Design review of the part built by this model. Coordinates are the model's own, in mm. A direction names the side the tool comes from. Give positions to 0.01 mm unless a question says otherwise; leave off trailing zeros. Loops run counter-clockwise (first coordinate to the right, second up) from the corner with the lowest first, then second, coordinate; pieces in that order, holes last. Notation, with made-up numbers: M 3.25,71.5 L 17.25,71.5 A32 ccw 17.25,107.5 Z; hole C -1,8 d7. An arc over 180 degrees is marked long. Use a Markdown table: item, result. Add a question column.
(1) Add section A-A, the plane x = 186. Give the boundary of the cut face in (y, z).
(2) Insertion check: pin 1 Ø1.5 at (x, y) = (199.5, -120.5) entering from +Z; pin 2 Ø5.5 at (x, z) = (2.5, -28.5) entering from +Y; pin 3 Ø1.5 at (x, y) = (51.5, -143) entering from +Z; pin 4 Ø6 at (y, z) = (-230, 15) entering from -X. Each pin has a flat end and moves straight along its axis. Give the tip position at first contact, or say it passes through.
(3) For faces 1 (the face through (138, -46.338, -1)), 2 (the face through (152, -41.338, -1)), list the 3-axis set-ups (+Z, -Z, +X, -X, +Y, -Y) from which the entire face can be reached by the end or side of a thin tool; tool diameter is ignored.
(4) For probe 1 along X at (y, z) = (-54.5, -0.5); probe 2 along Y at (x, z) = (119.5, -11.5); probe 3 along Y at (x, z) = (268, -5), list the stretches that pass through material, from the lowest coordinate up.
(5) Add section C-C, the plane y = -186.5. Give the boundary of the cut face in (x, z), then the cut area to 3 significant figures.
(6) Draft analysis for pull direction X (two halves, no side actions). For faces 3 (the face through (300, -204, -9)), 4 (the face through (147.9, -44.345, -22.148)), 5 (the face through (0, -204, -9)), 6 (the face through (275, -204, -11)), state which applies: pulls with the +X half, pulls with the -X half, needs draft (parallel to the pull), parting line crosses it, or undercut.
(7) Add section B-B, the plane y = -273.5. Give the boundary of the cut face in (x, z), then the cut area to 3 significant figures.
```python
from build123d import *

# Parameters (mm, degrees)
F1_DEPTH = 300
F2_T     = -5
F4_DEPTH = 25
F7_DEPTH = 5
F9_DEPTH = 300


# Not quite as in the source:
# - a feature of the source that left no trace in its solid (it failed there, or was rolled back) is left out
# - a feature names something its author has since deleted; it is built from what else it names


with BuildPart() as f1:
    # F0 (on Right) → F1 (new body)
    with BuildSketch(Plane.YZ):
        with BuildLine():
            ThreePointArc((-361.3383226016, -15), (-358.4093904135, -22.0710678119), (-351.3383226016, -25))
            Line((-351.3383226016, -25), (-51.3383226016, -25))
            ThreePointArc((-51.3383226016, -25), (-44.2672547897, -22.0710678119), (-41.3383226016, -15))
            Line((-41.3383226016, -15), (-41.3383226016, 13.3530771738))
            ThreePointArc((-41.3383226016, 13.3530771738), (-44.538361228, 20.6852341086), (-52.0904276652, 23.3247539622))
            Line((-52.0904276652, 23.3247539622), (-352.0904276652, 0.6975144458))
            ThreePointArc((-352.0904276652, 0.6975144458), (-358.6704795365, -2.474200969), (-361.3383226016, -9.2741623426))
            Line((-361.3383226016, -9.2741623426), (-361.3383226016, -15))
        make_face()
    extrude(amount=F1_DEPTH)

    # F2: a shell. OpenCascade refuses it in one call, so the cavity is built on its own and cut out:
    # the body offset inwards by the wall thickness, plus a prism from it out through each open face.
    f2_core = offset(f1.part, amount=F2_T, mode=Mode.PRIVATE)
    f2_exits = [f2_core.faces().sort_by_distance(p)[0] for p in [
        (150, -201.338323, -20),
    ]]
    add(f2_core, mode=Mode.SUBTRACT)
    extrude(f2_exits, amount=-F2_T, mode=Mode.SUBTRACT)

    # F4 (add): a face of the model
    f4_faces = [f1.faces().sort_by_distance(p)[0] for p in [
        (300, -183.9481701293, -5.8146709921),
    ]]
    extrude(f4_faces, amount=-F4_DEPTH)

    # F7 (add): faces of the model
    f7_faces = [f1.faces().sort_by_distance(p)[0] for p in [
        (2.5, -201.3383226016, -25),
        (287.5, -201.3383226016, -25),
    ]]
    extrude(f7_faces, amount=F7_DEPTH)

    # F0 (on Right) → F9 (cut)
    with BuildSketch(Plane.YZ):
        with BuildLine():
            ThreePointArc((-361.3383226016, -15), (-358.4093904135, -22.0710678119), (-351.3383226016, -25))
            Line((-351.3383226016, -25), (-51.3383226016, -25))
            ThreePointArc((-51.3383226016, -25), (-44.2672547897, -22.0710678119), (-41.3383226016, -15))
            Line((-41.3383226016, -15), (-41.3383226016, 13.3530771738))
            ThreePointArc((-41.3383226016, 13.3530771738), (-44.538361228, 20.6852341086), (-52.0904276652, 23.3247539622))
            Line((-52.0904276652, 23.3247539622), (-352.0904276652, 0.6975144458))
            ThreePointArc((-352.0904276652, 0.6975144458), (-358.6704795365, -2.474200969), (-361.3383226016, -9.2741623426))
            Line((-361.3383226016, -9.2741623426), (-361.3383226016, -15))
        make_face()
    extrude(amount=-F9_DEPTH, mode=Mode.SUBTRACT)


solid = f1.part
```
Established:
| question | item | result |
|---|---|---|
| 1 | outline | M -361.34,-15 A10 ccw -351.34,-25 L -351.34,-20 A5 cw -356.34,-15 L -356.34,-9.27 A5 cw -351.71,-4.29 L -51.71,18.34 A5 cw -46.34,13.35 L -46.34,-15 A5 cw -51.34,-20 L -51.34,-25 A10 ccw -41.34,-15 L -41.34,13.35 A10 ccw -52.09,23.32 L -352.09,0.7 A10 ccw -361.34,-9.27 Z |
| 2 | pin 1 | z = 18.22 |
| 2 | pin 2 | y = -51.34 |
| 2 | pin 3 | z = 16.52 |
| 2 | pin 4 | through |
| 3 | face 1 | none |
| 3 | face 2 | +Z, -Z, +X, -X, +Y |
| 4 | probe 1 | 0 to 5, 275 to 300 |
| 4 | probe 2 | -361.34 to -356.34, -46.34 to -41.34 |
| 4 | probe 3 | -360.38 to -353.93, -46.34 to -41.34 |
| 5 | outline | M 0,-30 L 5,-30 L 5,8.17 L 275,8.17 L 275,-30 L 300,-30 L 300,13.19 L 0,13.19 Z |
| 5 | area | 2,650 mm^2 |
| 6 | face 3 | pulls with the +X half |
| 6 | face 4 | needs draft |
| 6 | face 5 | pulls with the -X half |
| 6 | face 6 | undercut |
| 7 | outline | M 0,-30 L 5,-30 L 5,1.61 L 275,1.61 L 275,-30 L 300,-30 L 300,6.63 L 0,6.63 Z |
| 7 | area | 2,450 mm^2 |
